```python
from build123d import *

# Parameters (mm, degrees)
BOX_W         = 54
BOX_H         = 27
BOX_DEPTH     = 1
BOX001_W      = 10
BOX001_H      = 6
BOX001_DEPTH  = 1.1
CHAMFER_SIZE  = 1
ARRAY_X_COUNT = 5
ARRAY_X_PITCH = 11
ARRAY_Y_COUNT = 4
ARRAY_Y_PITCH = 7


with BuildPart() as cub:
    # Box → Box (new body)
    with BuildSketch(Plane.XY):
        with Locations((27, 13.5)):
            Rectangle(BOX_W, BOX_H)
    extrude(amount=BOX_DEPTH)


with BuildPart() as fusion:
    # Box001 → Box001 (new body)
    with BuildSketch(Plane(origin=(-13, 0, 0), x_dir=(1, 0, 0), z_dir=(0, 0, 1))):
        with Locations((5, 3)):
            Rectangle(BOX001_W, BOX001_H)
    extrude(amount=BOX001_DEPTH)

    # Chamfer
    chamfer_edges = [fusion.edges().sort_by_distance(p)[0] for p in [
        (-13, 3, 1.1),
        (-3, 3, 1.1),
        (-8, 0, 1.1),
        (-8, 6, 1.1),
    ]]
    chamfer(chamfer_edges, length=CHAMFER_SIZE)


with BuildPart() as fusion_1:
    # Chamfer placement: moved
    add(fusion.part.moved(Location((13.1, 0, 0.9))))

    # Array X: Fusion ×5


with BuildPart() as fusion_2:
    add(fusion_1.part)
    with Locations(*[(i * ARRAY_X_PITCH, 0, 0) for i in range(1, ARRAY_X_COUNT)]):
        add(fusion_1.part)

    # Array Y: Fusion ×4


with BuildPart() as fusion_3:
    add(fusion_2.part)
    with Locations(*[(0, i * ARRAY_Y_PITCH, 0) for i in range(1, ARRAY_Y_COUNT)]):
        add(fusion_2.part)

    # Fusion: union Cub
    add(cub.part)


solid = fusion_3.part
```
CAD build for the part. Positions are in the model's coordinates, mm. A direction names the side the tool comes from. Coordinates: 2 decimals unless noted, no trailing zeros. Order: outer loops, then holes, each group sorted by start corner. A loop starts at its lowest first (then second) coordinate and runs counter-clockwise, first axis right, second up. Notation, with made-up numbers: M 27,8.25 L 33,8.25 A23 cw 33,16.25 Z; hole C 30.25,-25.75 d6. An arc over 180 degrees is marked long. Write each question's results on one line, items separated by ' | '. Start each with the question number.
Q1. Which spindle directions (+Z, -Z, +X, -X, +Y, -Y) get a long thin tool onto all of the face, cutting with end or side? Do faces 4 (the flat face through (38, 14.5, 1.5)), 5 (the flat face through (33.6, 3, 1.5)), 6 (the flat face through (53.6, 24, 1.5)). Say none if no direction does.
Q2. Pull direction Y, two halves, no side cores. Call faces 1 (the flat face through (16, 26.5, 1.5)), 2 (the flat face through (38, 7.5, 1.5)), 3 (the flat face through (31.6, 24, 1.5)): +Y half, -Y half, draft (parallel to the pull), parting line (faces both ways), or undercut.
Q3. Cut at C-C (y = 4.25). List the corners of the cut face in (x, z), then the cut area to 3 significant figures.
Q4. Cut at A-A (x = 50.5). List the corners of the cut face in (y, z), then the cut area to 3 significant figures.
Q5. Drill centre lines: probe 1 along Y at (x, z) = (8.5, 1.65); probe 2 along X at (y, z) = (7.5, 1.4); probe 3 along Y at (x, z) = (20, 1.3). Where is each one in solid material? Low to high. Write a range as from..to.
Q6. Cut at B-B (z = 1.4). Count the separate pieces of the cut face and the enclosed holes in it, then the cut area to 3 significant figures.
Found:
1) face 4: +Z, +X, -X | face 5: +Z, +Y, -Y | face 6: +Z, +X, +Y, -Y
2) face 1: +Y half | face 2: undercut | face 3: draft
3) outline: M 0,0 L 54,0 L 54,0.9 L 54.1,0.9 L 54.1,1 L 53.1,2 L 45.1,2 L 44.1,1 L 43.1,1 L 42.1,2 L 34.1,2 L 33.1,1 L 32.1,1 L 31.1,2 L 23.1,2 L 22.1,1 L 21.1,1 L 20.1,2 L 12.1,2 L 11.1,1 L 10.1,1 L 9.1,2 L 1.1,2 L 0.1,1 L 0,1 Z | area: 99.0 mm²
4) outline: M 0,0 L 27,0 L 27,1 L 26,2 L 22,2 L 21,1 L 20,1 L 19,2 L 15,2 L 14,1 L 13,1 L 12,2 L 8,2 L 7,1 L 6,1 L 5,2 L 1,2 L 0,1 Z | area: 47.0 mm²
5) probe 1: 0.65..5.35, 7.65..12.35, 14.65..19.35, 21.65..26.35 | probe 2: 0.5..9.7, 11.5..20.7, 22.5..31.7, 33.5..42.7, 44.5..53.7 | probe 3: 0.3..5.7, 7.3..12.7, 14.3..19.7, 21.3..26.7
6) separate pieces: 20 | enclosed holes: 0 | area: 957 mm²
